Geometry: final body of the model. Coordinates: model frame, mm. A direction names the side the tool comes from. Give positions to 0.01 mm unless a question says otherwise; leave off trailing zeros. Order: outer loops, then holes, each group sorted by start corner. A loop starts at its lowest first (then second) coordinate and runs counter-clockwise, first axis right, second up. Notation, with made-up numbers: (-15.75, 12.25) -> (-11.75, 12.25) arc R17 ccw to (-11.75, 33.25) -> close; hole circle Ø9 at (-5.75, 6.25). An arc over 180 degrees is marked (long way). Answer in a Markdown table with one row per item. Add a question column.
Q1. Line query: line 1 along Y through (x, z) = (-307, 19); line 2 along X through (y, z) = (213, 19); line 3 along Z through (x, y) = (256, 213). Output: solid intervals per line, ascending. Write a range as from..to.
Q2. Pull-direction query (X, two-part tool) for faces 1 (the face through (-4, 214.2, 17)), 2 (the face through (-308, 104, 17)), 3 (the face through (306.5, 104, 17)), 4 (the face through (4, 212.7, 17)); classes: +X half, -X half, draft (parallel to the pull), parting line (faces both ways), or undercut.
Q3. Contact query for a flat-ended pin moving along its axis: P1, Ø3, axis at x = 229.5, z = 30.5, coming from the -Y side. Output: stop coordinate, or through.
Q4. Cut plane A-A on y = 168. Return the cut outline in (x, z), and give its area (3 significant figures).
Q5. Set-up query: faces 5 (the face through (-306.5, 107, 17)), 6 (the face through (308, 107, 17)). Return all of +Z, -Z, +X, -X, +Y, -Y with unobstructed straight access to the full face (end or side cutting, diameter ignored); none if empty.
Q6. Cut plane C-C on x = -217. Return the cut outline in (y, z).
Q7. Cut plane B-B on z = 26.5. Return the cut outline in (x, y).
from build123d import *

# Parameters (mm, degrees)
BASE_FLANGE1_DEPTH         = 34
SKETCH2_R                  = 2.05
CUT_EXTRUDE1_DEPTH         = 654.06480536
M6_CLEARANCE_HOLE1_D       = 6.4
FILLET1_R                  = 2
F_4_1_4_1_DIAMETER_HOLE1_D = 4.1


# Sheet-metal steps are written as plain solids
with BuildPart() as part:
    # Sketch1 → Base-Flange1 (new body)
    with BuildSketch(Plane.XY):
        with BuildLine():
            Line((-308, 0), (-308, 211.2))
            ThreePointArc((-308, 211.2), (-307.121320344, 213.321320344), (-305, 214.2))
            Line((-305, 214.2), (305, 214.2))
            ThreePointArc((305, 214.2), (307.121320344, 213.321320344), (308, 211.2))
            Line((308, 211.2), (308, 0))
            Line((308, 0), (306.5, 0))
            Line((306.5, 0), (306.5, 211.2))
            ThreePointArc((306.5, 211.2), (306.060660172, 212.260660172), (305, 212.7))
            Line((305, 212.7), (-305, 212.7))
            ThreePointArc((-305, 212.7), (-306.060660172, 212.260660172), (-306.5, 211.2))
            Line((-306.5, 211.2), (-306.5, 0))
            Line((-306.5, 0), (-308, 0))
        make_face()
    extrude(amount=BASE_FLANGE1_DEPTH)

    # Sketch2 → Cut-Extrude1 (cut, through all)
    with BuildSketch(Plane.ZY.offset(308)):
        with Locations((19, 12.2)):
            Circle(SKETCH2_R)
        with Locations((19, 75.7)):
            Circle(SKETCH2_R)
        with Locations((19, 139.2)):
            Circle(SKETCH2_R)
        with Locations((19, 202.7)):
            Circle(SKETCH2_R)
    extrude(amount=-CUT_EXTRUDE1_DEPTH, mode=Mode.SUBTRACT)

    # M6 Clearance Hole1 (through all)
    with Locations(Plane(origin=(0, 214.2, 0), x_dir=(1, 0, 0), z_dir=(0, 1, 0))):
        with Locations((-199.5, -12), (-169.5, -12)):
            m6_clearance_hole1 = Hole(M6_CLEARANCE_HOLE1_D / 2)

    # Fillet1
    fillet1_edges = [part.edges().sort_by_distance(p)[0] for p in [
        (-307.25, 0, 0),
        (307.25, 0, 0),
        (-307.25, 0, 34),
        (307.25, 0, 34),
    ]]
    fillet(fillet1_edges, radius=FILLET1_R)

    # Ø4.1 (4.1) Diameter Hole1 (through all)
    with Locations(Plane(origin=(0, 214.2, 0), x_dir=(1, 0, 0), z_dir=(0, 1, 0))):
        with Locations((-256.5, -19), (-120, -19), (0, -19), (120, -19), (256.5, -19)):
            Hole(F_4_1_4_1_DIAMETER_HOLE1_D / 2)

    # Mirror1: M6 Clearance Hole1 across Right Plane
    add(m6_clearance_hole1.mirror(Plane(origin=(0, 0, 0), x_dir=(0, 0, -1), z_dir=(1, 0, 0))), mode=Mode.SUBTRACT)


solid = part.part
Completed:
| question | item | result |
|---|---|---|
| 1 | line 1 | y = 0..10.15, 14.25..73.65, 77.75..137.15, 141.25..200.65, 204.75..213.44 |
| 1 | line 2 | x = -307.4..-258.55, -254.45..-122.05, -117.95..-2.05, 2.05..117.95, 122.05..254.45, 258.55..307.4 |
| 1 | line 3 | z = 0..17.01, 20.99..34 |
| 2 | face 1 | draft |
| 2 | face 2 | -X half |
| 2 | face 3 | undercut |
| 2 | face 4 | undercut |
| 3 | P1 | stops at y = 212.7 |
| 4 | outline | (-308, 0) -> (-306.5, 0) -> (-306.5, 34) -> (-308, 34) -> close; (306.5, 0) -> (308, 0) -> (308, 34) -> (306.5, 34) -> close |
| 4 | area | 102 mm² |
| 5 | face 5 | +Z, -Z, -Y |
| 5 | face 6 | +Z, -Z, +X, +Y, -Y |
| 6 | outline | (212.7, 0) -> (214.2, 0) -> (214.2, 34) -> (212.7, 34) -> close |
| 7 | outline | (-308, 0) -> (-306.5, 0) -> (-306.5, 211.2) arc R1.5 cw to (-305, 212.7) -> (305, 212.7) arc R1.5 cw to (306.5, 211.2) -> (306.5, 0) -> (308, 0) -> (308, 211.2) arc R3 ccw to (305, 214.2) -> (-305, 214.2) arc R3 ccw to (-308, 211.2) -> close |
